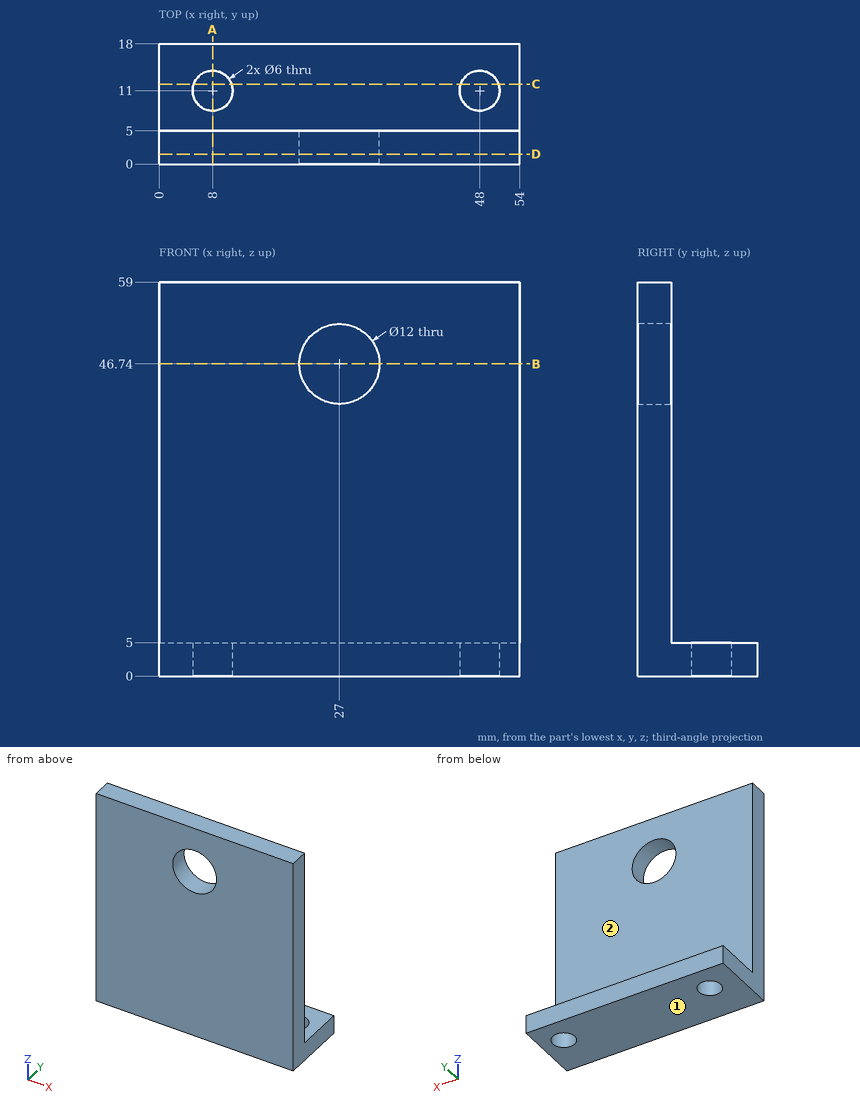
Job drawing, mm, ordinate dimensions from the low corner. One solid piece. A direction names the side the tool comes from. Round coordinates to 2 decimals unless told otherwise and drop trailing zeros. Order: outer loops, then holes, each group sorted by start corner. A loop starts at its lowest first (then second) coordinate and runs counter-clockwise, first axis right, second up. Notation, with made-up numbers: (72.25, 3) -> (122.25, 3) arc R18 ccw to (122.25, 34) -> close; hole circle Ø11 at (25.5, -29.5). An arc over 180 degrees is marked (long way). Answer in a Markdown table with one row per item.
1) Band-saw the part on A-A on x = 8. Give the cut face in (y, z).
Values:
| item | result |
|---|---|
| outline | (0, 0) -> (8, 0) -> (8, 5) -> (5, 5) -> (5, 59) -> (0, 59) -> close; (14, 0) -> (18, 0) -> (18, 5) -> (14, 5) -> close |
2) Wall check: L1, parallel to X at y = 11, z = 2.95; L2, parallel to Y at x = 8, z = 2; L3, parallel to X at y = 1.6, z = 46.74. Give the ranges that are in metal, low to high.
Values:
| item | result |
|---|---|
| L1 | 0 to 5, 11 to 45, 51 to 54 |
| L2 | 0 to 8, 14 to 18 |
| L3 | 0 to 21, 33 to 54 |
3) Pin check, flat tips, straight feed: P1, Ø2, axis at x = 17, z = 49.5, coming from the -Y side; P2, Ø14, axis at x = 27, z = 46.74, coming from the +Y side. Stop position of each tip, or through.
Values:
| item | result |
|---|---|
| P1 | y = 0 |
| P2 | y = 5 |
4) Band-saw the part on D-D on y = 1.5. Give the cut face in (x, z).
Values:
| item | result |
|---|---|
| outline | (0, 0) -> (54, 0) -> (54, 59) -> (0, 59) -> close; hole circle Ø12 at (27, 46.74) |
5) Band-saw the part on B-B on z = 46.74. Give the cut face in (x, y).
Values:
| item | result |
|---|---|
| outline | (0, 0) -> (21, 0) -> (21, 5) -> (0, 5) -> close; (33, 0) -> (54, 0) -> (54, 5) -> (33, 5) -> close |
6) Which spindle directions (+Z, -Z, +X, -X, +Y, -Y) get a long thin tool onto all of the face, cutting with end or side? Do the marked faces 1 and 2. Say none if no direction does.
Values:
| item | result |
|---|---|
| face 1 | -Z, +X, -X, +Y, -Y |
| face 2 | +Z, +X, -X, +Y |
7) Band-saw the part on C-C on y = 12. Give the cut face in (x, z), and give its area (3 significant figures).
Values:
| item | result |
|---|---|
| outline | (0, 0) -> (5.17, 0) -> (5.17, 5) -> (0, 5) -> close; (10.83, 0) -> (45.17, 0) -> (45.17, 5) -> (10.83, 5) -> close; (50.83, 0) -> (54, 0) -> (54, 5) -> (50.83, 5) -> close |
| area | 213 mm2 |
